from build123d import *

# Parameters (mm, degrees)
F0_R     = 1.1
F0_R_2   = 1.075
F1_DEPTH = 2.6


with BuildPart() as f1:
    # F0 (on Top) → F1 (new body)
    with BuildSketch(Plane.XY):
        with BuildLine():
            ThreePointArc((-4.746486, 4.808329), (-5.079824, 1.124576), (-1.822392, 2.876799))
            ThreePointArc((-1.822392, 2.876799), (-2.614969, 4.520158), (-4.394433, 4.923045))
            ThreePointArc((-4.394433, 4.923045), (-4.572993, 4.873462), (-4.746486, 4.808329))
        make_face()
        with Locations((-3.922381, 2.876799)):
            Circle(F0_R, mode=Mode.SUBTRACT)
        with BuildLine():
            ThreePointArc((-4.394433, 4.923045), (-2.614969, 4.520158), (-1.822392, 2.876799))
            ThreePointArc((-1.822392, 2.876799), (-5.079824, 1.124576), (-4.746486, 4.808329))
            Line((-4.746486, 4.808329), (-15.782993, 0.099507))
            ThreePointArc((-15.782993, 0.099507), (-13.659897, -0.09261), (-12.65002, -1.97))
            ThreePointArc((-12.65002, -1.97), (-12.802118, -2.78321), (-13.237851, -3.486475))
            Line((-13.237851, -3.486475), (-12.155538, -2.30018))
            Line((-12.155538, -2.30018), (5.849769, 3.333367))
            Line((5.849769, 3.333367), (18.365619, 3.333367))
            Line((18.365619, 3.333367), (23.356251, 2.544399))
            ThreePointArc((23.356251, 2.544399), (22.108876, 4.260224), (23.824702, 5.507599))
            Line((23.824702, 5.507599), (8.583845, 7.917022))
            Line((8.583845, 7.917022), (-4.394433, 4.923045))
        make_face()
        with BuildLine():
            ThreePointArc((-12.65002, -1.97), (-13.659897, -0.09261), (-15.782993, 0.099507))
            ThreePointArc((-15.782993, 0.099507), (-16.73485, -3.272267), (-13.237851, -3.486475))
            ThreePointArc((-13.237851, -3.486475), (-12.802118, -2.78321), (-12.65002, -1.97))
        make_face()
        with Locations((-14.90002, -1.97)):
            Circle(F0_R, mode=Mode.SUBTRACT)
        with BuildLine():
            ThreePointArc((25.090476, 4.025999), (24.730945, 5.000335), (23.824702, 5.507599))
            ThreePointArc((23.824702, 5.507599), (22.108876, 4.260224), (23.356251, 2.544399))
            ThreePointArc((23.356251, 2.544399), (24.564812, 2.88553), (25.090476, 4.025999))
        make_face()
        with Locations((23.590476, 4.025999)):
            Circle(F0_R_2, mode=Mode.SUBTRACT)
    extrude(amount=F1_DEPTH)


solid = f1.part
Part model, mm, in its own coordinate system. A direction names the side the tool comes from. Coordinates: 2 decimals unless noted, no trailing zeros. Loops run counter-clockwise (first coordinate to the right, second up) from the corner with the lowest first, then second, coordinate; pieces in that order, holes last. Notation, with made-up numbers: (22, -4) -> (38, -4) arc R30 cw to (38, 19) -> close; hole circle Ø4 at (62.5, 7.25). An arc over 180 degrees is marked (long way). Use a Markdown table: item, result. Add a question column.
Item 1: Flat gauge pin, fed straight in: P1, Ø2, axis at x = 4.5, y = 0, coming from the +Z side. Where does the tip first touch, or does it go through?
Item 2: Which spindle directions (+Z, -Z, +X, -X, +Y, -Y) get a long thin tool onto all of the face, cutting with end or side? Do faces 5 (the flat face through (16.311, 6.695, 1.282)), 6 (the flat face through (20.826, 2.944, 1.282)). Say none if no direction does.
Item 3: Band-saw the part on A-A on z = 1.4. Give the number of separate pieces and of enclosed holes in the cut face, plus the area to 3 significant figures.
Item 4: Pull direction Y, two halves, no side cores. Call faces 1 (the cylindrical face through (-2.873, 3.207, 1.282)), 2 (the flat face through (-12.704, -2.902, 1.282)), 3 (the cylindrical face through (-13.884, -2.391, 1.282)), 4 (the cylindrical face through (-16.767, -3.226, 1.282)): +Y half, -Y half, draft (parallel to the pull), parting line (faces both ways), or undercut.
Item 5: Band-saw the part on C-C on x = -10.5. Write the cut outline in (y, z), plus the area to 3 significant figures.
Item 6: Band-saw the part on B-B on x = 14. Write the cut outline in (y, z), plus the area to 3 significant figures.
Item 7: Probe probe 1 along Y at (x, z) = (-15, 1.6); probe 2 along Y at (x, z) = (19.5, 0.15); probe 3 along Y at (x, z) = (9, 0.4). List the from-to ranges inside material, lowest first.
Geometry says:
| question | item | result |
|---|---|---|
| 1 | P1 | through |
| 2 | face 5 | +Z, -Z, +X, +Y |
| 2 | face 6 | +Z, -Z, -Y |
| 3 | separate pieces | 1 |
| 3 | enclosed holes | 3 |
| 3 | area | 157 mm² |
| 4 | face 1 | undercut |
| 4 | face 2 | -Y half |
| 4 | face 3 | undercut |
| 4 | face 4 | parting line |
| 5 | outline | (-1.78, 0) -> (2.35, 0) -> (2.35, 2.6) -> (-1.78, 2.6) -> close |
| 5 | area | 10.8 mm² |
| 6 | outline | (3.33, 0) -> (7.06, 0) -> (7.06, 2.6) -> (3.33, 2.6) -> close |
| 6 | area | 9.69 mm² |
| 7 | probe 1 | -4.22 to -3.07, -0.87 to 0.43 |
| 7 | probe 2 | 3.15 to 6.19 |
| 7 | probe 3 | 3.33 to 7.85 |
